For this review, use the dimensioned drawing (mm, ordinates from the lowest corner) and the shaded views. A direction names the side the tool comes from. Give positions to 0.01 mm unless a question says otherwise; leave off trailing zeros. Order: outer loops, then holes, each group sorted by start corner. A loop starts at its lowest first (then second) coordinate and runs counter-clockwise, first axis right, second up. Notation, with made-up numbers: M 34,46.25 L 78,46.25 A34 ccw 78,76.25 Z; hole C 54.5,-24 d1. An arc over 180 degrees is marked long. Use CSV: the item, a comma, the result in double quotes. Start each with the question number.
(1) Consider section C-C (y = 3.25). Write out the cut boundary in (x, z), and give its area (3 significant figures).
(2) Draft analysis for pull direction Z (two halves, no side actions). For the marked faces 6, 7, 8 and 9, state which applies: pulls with the +Z half, pulls with the -Z half, needs draft (parallel to the pull), parting line crosses it, or undercut.
(3) Consider section B-B (x = 9.5). Write out the cut boundary in (y, z), and give its area (3 significant figures).
(4) Clearance check with flat-ended pins moving along their axes: P1, Ø6, axis at y = 22, z = 10, coming from the -X side; P2, Ø2, axis at y = 10, z = 4.5, coming from the -X side; P3, Ø1, axis at x = 4.5, z = 4, coming from the +Y side. State where each tip first meets the part, or that it passes through.
(5) Tool access review of the marked faces 1, 2, 3, 4 and 5: name each direction out of +Z, -Z, +X, -X, +Y, -Y from which nothing blocks a thin tool from reaching the whole face with its end or side.
(6) Wall thickness on L1, parallel to Y at x = 12.75, z = 1; L2, parallel to Z at x = 24.25, y = 11; L3, parallel to X at y = 15.5, z = 8.75: over which ranges is each line inside the solid? List them lowest first. Write a range as from..to.
(7) Consider section A-A (y = 14.75). Write out the cut boundary in (x, z), and give its area (3 significant figures).
(8) Consider section D-D (x = 18). Write out the cut boundary in (y, z), and give its area (3 significant figures).
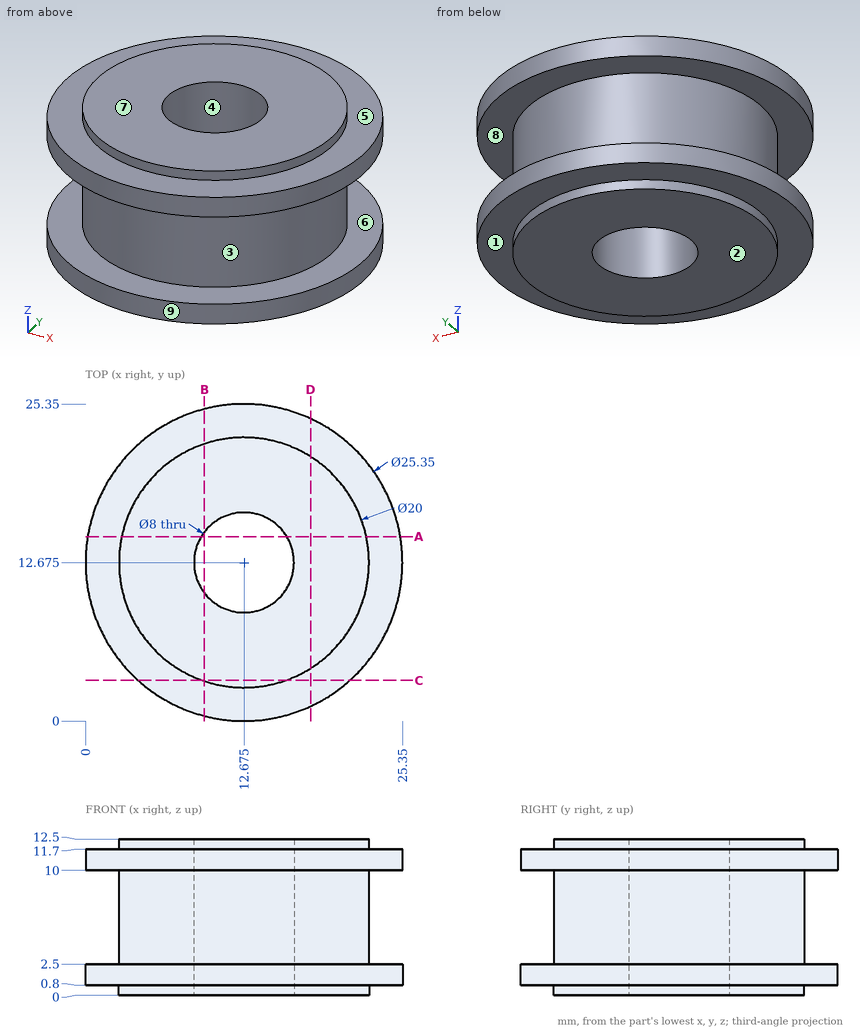
Check result:
1,outline,"M 4.2,0.8 L 9.33,0.8 L 9.33,0 L 16.02,0 L 16.02,0.8 L 21.15,0.8 L 21.15,2.5 L 16.02,2.5 L 16.02,10 L 21.15,10 L 21.15,11.7 L 16.02,11.7 L 16.02,12.5 L 9.33,12.5 L 9.33,11.7 L 4.2,11.7 L 4.2,10 L 9.33,10 L 9.33,2.5 L 4.2,2.5 Z"
1,area,"118 mm^2"
2,face 6,"undercut"
2,face 7,"pulls with the +Z half"
2,face 8,"undercut"
2,face 9,"needs draft"
3,outline,"M 0.4,0.8 L 3.19,0.8 L 3.19,0 L 10.24,0 L 10.24,12.5 L 3.19,12.5 L 3.19,11.7 L 0.4,11.7 L 0.4,10 L 3.19,10 L 3.19,2.5 L 0.4,2.5 Z; M 15.11,0 L 22.16,0 L 22.16,0.8 L 24.95,0.8 L 24.95,2.5 L 22.16,2.5 L 22.16,10 L 24.95,10 L 24.95,11.7 L 22.16,11.7 L 22.16,12.5 L 15.11,12.5 Z"
3,area,"195 mm^2"
4,P1,"stops at x = 1.69"
4,P2,"stops at x = 2.82"
4,P3,"stops at y = 19.09"
5,face 1,"-Z"
5,face 2,"-Z, +X, -X, +Y, -Y"
5,face 3,"none"
5,face 4,"+Z, -Z"
5,face 5,"+Z"
6,L1,"y = 0..8.68, 16.67..25.35"
6,L2,"z = 0.8..2.5, 10..11.7"
6,L3,"x = 3.08..9.84, 15.51..22.27"
7,outline,"M 0.17,0.8 L 2.89,0.8 L 2.89,0 L 9.26,0 L 9.26,12.5 L 2.89,12.5 L 2.89,11.7 L 0.17,11.7 L 0.17,10 L 2.89,10 L 2.89,2.5 L 0.17,2.5 Z; M 16.09,0 L 22.46,0 L 22.46,0.8 L 25.18,0.8 L 25.18,2.5 L 22.46,2.5 L 22.46,10 L 25.18,10 L 25.18,11.7 L 22.46,11.7 L 22.46,12.5 L 16.09,12.5 Z"
7,area,"178 mm^2"
8,outline,"M 1.17,0.8 L 4.21,0.8 L 4.21,0 L 21.14,0 L 21.14,0.8 L 24.18,0.8 L 24.18,2.5 L 21.14,2.5 L 21.14,10 L 24.18,10 L 24.18,11.7 L 21.14,11.7 L 21.14,12.5 L 4.21,12.5 L 4.21,11.7 L 1.17,11.7 L 1.17,10 L 4.21,10 L 4.21,2.5 L 1.17,2.5 Z"
8,area,"232 mm^2"
